Design review of the part built by this model. Coordinates are the model's own, in mm. A direction names the side the tool comes from. Give positions to 0.01 mm unless a question says otherwise; leave off trailing zeros. Put each result on its own line as item: value. Start each with the question number.
from build123d import *

# Parameters (mm, degrees)
EXTRUDE_1_DEPTH = 2.5
FILLET_1_R      = 2


with BuildPart() as part:
    # 草圖1 → 填料-伸長1 (new, symmetric)
    with BuildSketch(Plane.XY):
        with BuildLine():
            Line((-25, 2), (-23, 0))
            Line((-23, 0), (23, 0))
            Line((23, 0), (25, 2))
            Line((25, 2), (25, 4))
            ThreePointArc((25, 4), (24.292893219, 5.707106781), (26, 5))
            Line((26, 5), (35, 5))
            Line((35, 5), (35, 47.5))
            Line((35, 47.5), (23, 47.5))
            Line((23, 47.5), (23, 52.5))
            Line((23, 52.5), (35, 52.5))
            Line((35, 52.5), (35, 87.5))
            Line((35, 87.5), (23, 87.5))
            Line((23, 87.5), (23, 92.5))
            Line((23, 92.5), (35, 92.5))
            Line((35, 92.5), (35, 127.5))
            Line((35, 127.5), (23, 127.5))
            Line((23, 127.5), (23, 132.5))
            Line((23, 132.5), (35, 132.5))
            Line((35, 132.5), (35, 167.5))
            Line((35, 167.5), (23, 167.5))
            Line((23, 167.5), (23, 172.5))
            Line((23, 172.5), (35, 172.5))
            Line((35, 172.5), (35, 207.5))
            Line((35, 207.5), (23, 207.5))
            Line((23, 207.5), (23, 212.5))
            Line((23, 212.5), (35, 212.5))
            Line((35, 212.5), (35, 255))
            Line((35, 255), (26, 255))
            ThreePointArc((26, 255), (24.292893219, 254.292893219), (25, 256))
            Line((25, 256), (25, 258))
            Line((25, 258), (23, 260))
            Line((23, 260), (-23, 260))
            Line((-23, 260), (-25, 258))
            Line((-25, 258), (-25, 256))
            ThreePointArc((-25, 256), (-24.292893219, 254.292893219), (-26, 255))
            Line((-26, 255), (-35, 255))
            Line((-35, 255), (-35, 5))
            Line((-35, 5), (-26, 5))
            ThreePointArc((-26, 5), (-24.292893219, 5.707106781), (-25, 4))
            Line((-25, 4), (-25, 2))
        make_face()
    extrude(amount=EXTRUDE_1_DEPTH, both=True)

    # 圓角1
    fillet_1_edges = [part.edges().sort_by_distance(p)[0] for p in [
        (35, 47.5, 0),
        (23, 47.5, 0),
        (23, 52.5, 0),
        (35, 52.5, 0),
        (35, 87.5, 0),
        (23, 87.5, 0),
        (23, 92.5, 0),
        (35, 92.5, 0),
        (35, 127.5, 0),
        (23, 127.5, 0),
        (23, 132.5, 0),
        (35, 132.5, 0),
        (35, 167.5, 0),
        (23, 167.5, 0),
        (23, 172.5, 0),
        (35, 172.5, 0),
        (35, 207.5, 0),
        (23, 207.5, 0),
        (23, 212.5, 0),
        (35, 212.5, 0),
    ]]
    fillet(fillet_1_edges, radius=FILLET_1_R)


solid = part.part
1. Insertion check: pin 1 (1.6 mm diameter, centred on x = 25, y = 255, fed in from +Z); pin 2 (2.5 mm diameter, centred on x = 30.5, z = 0.5, fed in from +Y); pin 3 (0.5 mm diameter, centred on y = 170, z = 1, fed in from +X); pin 4 (1.5 mm diameter, centred on x = -10, z = -0.5, fed in from -Y). Each pin has a flat end and moves straight along its axis. Give the tip position at first contact, or say it passes through.
2. Machinability: for faces 1 (the flat face through (31, 255, 0)), 2 (the flat face through (-30, 255, 0)), 3 (the flat face through (29, 167.5, 0)), which of the approach directions +Z, -Z, +X, -X, +Y, -Y give a long, thin tool a straight path to every point of the face, cutting with its end or side? Answer none if there is none.
3. To check wall thickness, follow probe 1 along Y at (x, z) = (-31, -0.35); probe 2 along X at (y, z) = (214, 0.9). State the ranges of each line that lie inside material, in increasing order.
4. The part is to be moulded in two halves that separate along Y. For faces 4 (the flat face through (-31, 5, 0)), 5 (the flat face through (29, 87.5, 0)), 6 (the flat face through (35, 70, 0)), say which applies: +Y half, -Y half, draft (parallel to the pull), parting line (faces both ways), or undercut.
Returned:
1. pin 1: passes through
1. pin 2: stops at y = 255
1. pin 3: stops at x = 23
1. pin 4: stops at y = 0
2. face 1: +Z, -Z, +X, +Y
2. face 2: +Z, -Z, -X, +Y
2. face 3: +Z, -Z, +X
3. probe 1: y = 5 to 255
3. probe 2: x = -35 to 34.94
4. face 4: -Y half
4. face 5: undercut
4. face 6: draft
